CAD build for the part. Positions are in the model's coordinates, mm. Coordinates: 2 decimals unless noted, no trailing zeros. Order: outer loops, then holes, each group sorted by start corner. A loop starts at its lowest first (then second) coordinate and runs counter-clockwise, first axis right, second up. Notation, with made-up numbers: (34.5, -3.5) - (73.5, -3.5) arc R5 cw to (73.5, 1.5) - close; hole circle Ø6 at (14.25, -29). An arc over 180 degrees is marked (long way). Return JSON: item names as keys, results as strings.
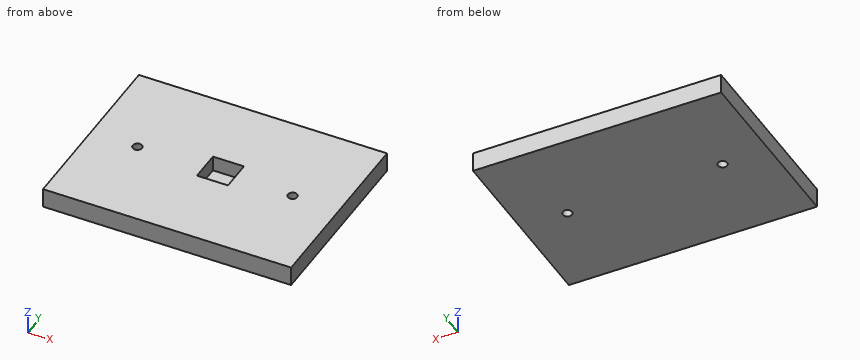
from build123d import *

# Parameters (mm, degrees)
SKETCH1_W           = 159.999934
SKETCH1_H           = 120
SKETCH1_R           = 3
BOSS_EXTRUDE1_DEPTH = 12.7
SKETCH3_W           = 20
SKETCH3_H           = 20
CUT_EXTRUDE3_DEPTH  = 10


with BuildPart() as part:
    # Sketch1 → Boss-Extrude1 (new body)
    with BuildSketch(Plane.XY):
        with Locations((47.542890143, -13.714285714)):
            Rectangle(SKETCH1_W, SKETCH1_H)
        with Locations(Location((97.542231184, -13.714285714, 0), (0, 0, 180))):
            Circle(SKETCH1_R, mode=Mode.SUBTRACT)
        with Locations(Location((-2.485927723, -13.714285714, 0), (0, 0, 180))):
            Circle(SKETCH1_R, mode=Mode.SUBTRACT)
    extrude(amount=BOSS_EXTRUDE1_DEPTH)

    # Sketch3 → Cut-Extrude3 (cut)
    with BuildSketch(Plane.XY.offset(12.7)):
        with Locations((50.220438118, -12.079110468)):
            Rectangle(SKETCH3_W, SKETCH3_H)
    extrude(amount=-CUT_EXTRUDE3_DEPTH, mode=Mode.SUBTRACT)


solid = part.part
Item 1: Band-saw the part on A-A, the plane x = 48. List the corners of the cut face in (y, z).
Findings below:
{"outline": "(-73.71, 0) - (46.29, 0) - (46.29, 12.7) - (-2.08, 12.7) - (-2.08, 2.7) - (-22.08, 2.7) - (-22.08, 12.7) - (-73.71, 12.7) - close"}
Item 2: Drop a flat-ended pin along its axis: P1, Ø10, axis at x = 48, y = -9.5, coming from the +Z side. Give the stop position or say it passes through.
Findings below:
{"P1": "stops at z = 2.7"}
Item 3: Band-saw the part on B-B, the plane z = 5.5. List the corners of the cut face in (x, y).
Findings below:
{"outline": "(-32.46, -73.71) - (127.54, -73.71) - (127.54, 46.29) - (-32.46, 46.29) - close; hole circle Ø6 at (-2.49, -13.71); hole (40.22, -22.08) - (60.22, -22.08) - (60.22, -2.08) - (40.22, -2.08) - close; hole circle Ø6 at (97.54, -13.71)"}
Item 4: Wall check: L1, parallel to Y at x = 51, z = 7.75; L2, parallel to X at y = -3.5, z = 5.5; L3, parallel to Z at x = 53.5, y = -5.5. Give the ranges that are in metal, low to high. Write a range as [from, to].
Findings below:
{"L1": "y = [-73.71, -22.08], [-2.08, 46.29]", "L2": "x = [-32.46, 40.22], [60.22, 127.54]", "L3": "z = [0, 2.7]"}
